from build123d import *

# Parameters (mm, degrees)
SKETCH1_R            = 9.525
EXTRUDE1_DEPTH       = 19.05
CHAMFER1_SIZE        = 0.4064
TRUNCATED_DEPTH      = 20.05
TRUNCATED_DEPTH_BACK = 20.05
RECESSED_DEPTH       = 0.127
SKETCH4_R            = 2.5527
THREADED_DEPTH       = 6.35
CHAMFER2_SIZE        = 0.6223


with BuildPart() as part:
    # Sketch1 → Extrude1 (new body, symmetric)
    with BuildSketch(Plane.XY):
        Circle(SKETCH1_R)
    extrude(amount=EXTRUDE1_DEPTH, both=True)

    # Chamfer1
    chamfer1_edges = [part.edges().sort_by_distance(p)[0] for p in [
        (-9.525, 0, -19.05),
        (-9.525, 0, 19.05),
    ]]
    chamfer(chamfer1_edges, length=CHAMFER1_SIZE)

    # Sketch2 → Truncated (cut, two sides)
    with BuildSketch(Plane.XY) as truncated_sk:
        with BuildLine():
            Line((-8.980256121, -3.175), (8.980256121, -3.175))
            ThreePointArc((8.980256121, -3.175), (0, -9.525), (-8.980256121, -3.175))
        make_face()
    extrude(amount=TRUNCATED_DEPTH, mode=Mode.SUBTRACT)
    extrude(truncated_sk.sketch, amount=-TRUNCATED_DEPTH_BACK, mode=Mode.SUBTRACT)

    # Sketch3 → Recessed (cut)
    with BuildSketch(Plane.XZ.offset(3.175)):
        with BuildLine():
            Line((6.091006121, 16.66875), (-6.091006121, 16.66875))
            ThreePointArc((-6.091006121, 16.66875), (-6.450216366, 16.519960245), (-6.599006121, 16.16075))
            Line((-6.599006121, 16.16075), (-6.599006121, -16.16075))
            ThreePointArc((-6.599006121, -16.16075), (-6.450216366, -16.519960245), (-6.091006121, -16.66875))
            Line((-6.091006121, -16.66875), (6.091006121, -16.66875))
            ThreePointArc((6.091006121, -16.66875), (6.450216366, -16.519960245), (6.599006121, -16.16075))
            Line((6.599006121, -16.16075), (6.599006121, 16.16075))
            ThreePointArc((6.599006121, 16.16075), (6.450216366, 16.519960245), (6.091006121, 16.66875))
        make_face()
    extrude(amount=-RECESSED_DEPTH, mode=Mode.SUBTRACT)

    # Sketch4 → Threaded (cut)
    with BuildSketch(Plane.XZ.offset(3.175)):
        with Locations(Location((0, 12.7, 0), (0, 0, 270))):  # turned: the seam where the file's is
            Circle(SKETCH4_R)
        with Locations(Location((0, -12.7, 0), (0, 0, 270))):  # turned: the seam where the file's is
            Circle(SKETCH4_R)
    extrude(amount=-THREADED_DEPTH, mode=Mode.SUBTRACT)

    # Chamfer2
    chamfer2_edges = [part.edges().sort_by_distance(p)[0] for p in [
        (0, -3.048, 15.2527),
        (0, -3.048, -10.1473),
    ]]
    chamfer(chamfer2_edges, length=CHAMFER2_SIZE)


solid = part.part
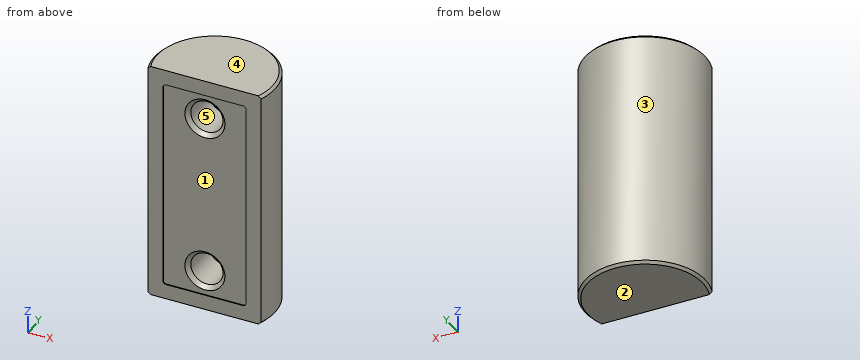
For this review, take the finished solid that the model builds, in its own axes (mm). Face numbers are marked on the shaded views. A direction names the side the tool comes from. Give positions to 0.01 mm unless a question says otherwise; leave off trailing zeros. Order: outer loops, then holes, each group sorted by start corner. A loop starts at its lowest first (then second) coordinate and runs counter-clockwise, first axis right, second up. Notation, with made-up numbers: (33.5, 1) - (38.5, 1) arc R11 cw to (38.5, 18) - close; hole circle Ø7 at (80.5, 49). An arc over 180 degrees is marked (long way). Answer as a JSON object with one key per item and string values. Group by question number.
Item 1: Take a section at D-D on z = -3. Give the boundary of the cut face in (x, y) (3 decimals), and give its area (3 significant figures).
Item 2: Take a section at A-A on y = 0. Give the boundary of the cut face in (x, z) (3 decimals), and give its area (3 significant figures).
Item 3: Take a section at B-B on z = -12.7. Give the boundary of the cut face in (x, y) (3 decimals), and give its area (3 significant figures).
Item 4: Wall thickness on line 1 along X through (y, z) = (-0.25, 12.7); line 2 along Z through (x, y) = (1.5, -1); line 3 along X through (y, z) = (1.55, 12.7): over which ranges is each line inside the solid? List them lowest first.
Item 5: Clearance check with flat-ended pins moving along their axes: pin 1 Ø1.5 at (x, z) = (-1, 12.5) entering from -Y (3 decimals); pin 2 Ø1 at (y, z) = (-1, 1) entering from +X; pin 3 Ø1.5 at (y, z) = (4, -14.5) entering from +X. State where each tip first meets the part, or that it passes through.
Item 6: Draft analysis for pull direction X (two halves, no side actions). For the marked faces 1, 2 and 3, state which applies: pulls with the +X half, pulls with the -X half, needs draft (parallel to the pull), parting line crosses it, or undercut.
Item 7: Take a section at C-C on x = 0. Give the boundary of the cut face in (y, z) (3 decimals), and give its area (3 significant figures).
Item 8: Machinability: for the marked faces 4 and 5, which of the approach directions +Z, -Z, +X, -X, +Y, -Y give a long, thin tool a straight path to every point of the face, cutting with its end or side? Answer none if there is none.
Reported:
{
 "1": {"outline": "(-8.98, -3.175) - (-6.599, -3.175) - (-6.599, -3.048) - (6.599, -3.048) - (6.599, -3.175) - (8.98, -3.175) arc R9.525 ccw (long way) to start", "area": "200 mm^2"},
 "2": {"outline": "(-9.525, -18.644) - (-9.119, -19.05) - (9.119, -19.05) - (9.525, -18.644) - (9.525, 18.644) - (9.119, 19.05) - (-9.119, 19.05) - (-9.525, 18.644) - close; hole circle Ø5.105 at (0, -12.7); hole circle Ø5.105 at (0, 12.7)", "area": "685 mm^2"},
 "3": {"outline": "(-8.98, -3.175) - (-6.599, -3.175) - (-6.599, -3.048) - (-3.175, -3.048) - (-2.553, -2.426) - (-2.553, 3.175) - (2.553, 3.175) - (2.553, -2.426) - (3.175, -3.048) - (6.599, -3.048) - (6.599, -3.175) - (8.98, -3.175) arc R9.525 ccw (long way) to start", "area": "168 mm^2"},
 "4": {"line 1": "-9.52 to -2.55, 2.55 to 9.52", "line 2": "-19.05 to -14.77, -10.63 to 10.63, 14.77 to 19.05", "line 3": "-9.4 to -2.55, 2.55 to 9.4"},
 "5": {"pin 1": "y = 3.175", "pin 2": "x = 9.51", "pin 3": "x = 8.95"},
 "6": {"face 1": "undercut", "face 2": "needs draft", "face 3": "parting line crosses it"},
 "7": {"outline": "(-3.175, -19.05) - (9.119, -19.05) - (9.525, -18.644) - (9.525, 18.644) - (9.119, 19.05) - (-3.175, 19.05) - (-3.175, 16.669) - (-3.048, 16.669) - (-3.048, 15.875) - (-2.426, 15.253) - (3.175, 15.253) - (3.175, 10.147) - (-2.426, 10.147) - (-3.048, 9.525) - (-3.048, -9.525) - (-2.426, -10.147) - (3.175, -10.147) - (3.175, -15.253) - (-2.426, -15.253) - (-3.048, -15.875) - (-3.048, -16.669) - (-3.175, -16.669) - close", "area": "415 mm^2"},
 "8": {"face 4": "+Z, +X, -X, +Y, -Y", "face 5": "-Y"}
}
